Read the model definition and answer for the solid it produces. Units are mm, in the model's axes. Face numbers are marked on the shaded views. A direction names the side the tool comes from. Coordinates: 2 decimals unless noted, no trailing zeros. Write each loop counter-clockwise with the first axis right and the second up, starting at its lowest first coordinate (ties: lowest second). Pieces come first, ordered by that corner, then holes.
Item 1: A tool of negligible diameter and unlimited length cuts with its end or side. For the marked faces 4, 5 and 6, from which of +Z, -Z, +X, -X, +Y, -Y can it reach the whole face along a straight path? Write none if from no direction.
Item 2: Section D-D (z = -4) is taken. Give the vertices of the cut face in (x, y), then the cut area to 3 significant figures.
Item 3: Section B-B (y = 5.25) is taken. Give the vertices of the cut face in (x, z), then the cut area to 3 significant figures.
Item 4: Section C-C (x = 0) is taken. Give the vertices of the cut face in (y, z), then the cut area to 3 significant figures.
Item 5: Section A-A (z = -7) is taken. Give the vertices of the cut face in (x, y).
Item 6: Straight lines are drawn through the part: probe 1 along Z at (x, y) = (1.25, 8.5); probe 2 along X at (y, z) = (0, -6.1); probe 3 along Y at (x, z) = (0, -6.6). For each, find the intervals that lie inside material, in ascending order.
Item 7: Each of these flat-tipped pins is pushed along its axis until it touches: P1, Ø2, axis at x = 4, z = 0, coming from the +Y side; P2, Ø4, axis at y = -4, z = -6.5, coming from the -X side; P3, Ø1.5, axis at x = 7.5, z = -2, coming from the -Y side; P4, Ø1.5, axis at x = -0.5, y = -0.5, coming from the -Z side. Where does it stop, or does it pass through?
Item 8: Determine the mould class of the marked faces 1, 2 and 3 for opening direction X: released by +X, released by -X, zero draft, split by the parting line, or undercut.
from build123d import *

# Parameters (mm, degrees)
F0_R     = 10.5
F0_R_2   = 9
F0_R_3   = 3
F1_DEPTH = 1
F2_DEPTH = 5
F3_DEPTH = 0.1
F4_DEPTH = 0.1
F5_R     = 9
F6_DEPTH = 0.1
F7_R     = 1.5
F8_DEPTH = 4.5


with BuildPart() as f1:
    # F0 (on Top) → F1 (new body)
    with BuildSketch(Plane.XY):
        Circle(F0_R)
        Circle(F0_R_2, mode=Mode.SUBTRACT)
        Circle(F0_R_2)
        Circle(F0_R_3, mode=Mode.SUBTRACT)
        Circle(F0_R_3)
    extrude(amount=F1_DEPTH)

    # F0 (on Top) → F2 (join)
    with BuildSketch(Plane.XY):
        Circle(F0_R_3)
    extrude(amount=-F2_DEPTH)

    # F0 (on Top) → F3 (join)
    with BuildSketch(Plane.XY):
        Circle(F0_R_2)
        Circle(F0_R_3, mode=Mode.SUBTRACT)
    extrude(amount=F3_DEPTH)

    # F0 (on Top) → F4 (join)
    with BuildSketch(Plane.XY):
        Circle(F0_R_2)
        Circle(F0_R_3, mode=Mode.SUBTRACT)
    extrude(amount=-F4_DEPTH)

    # F5 (on face) → F6 (join)
    with BuildSketch(Plane.XY.offset(1)):
        Circle(F5_R)
    extrude(amount=F6_DEPTH)

    # F7 (on face) → F8 (join)
    with BuildSketch(Plane(origin=(0, 0, -5), x_dir=(1, 0, 0), z_dir=(0, 0, -1))):
        Polygon((1.668331337, -2.4933251994), (2.9934486311, 0.1981547201), (1.325117294, 2.6914799195), (-1.668331337, 2.4933251994), (-2.9934486311, -0.1981547201), (-1.325117294, -2.6914799195), align=None)
        Circle(F7_R, mode=Mode.SUBTRACT)
    extrude(amount=F8_DEPTH)


solid = f1.part
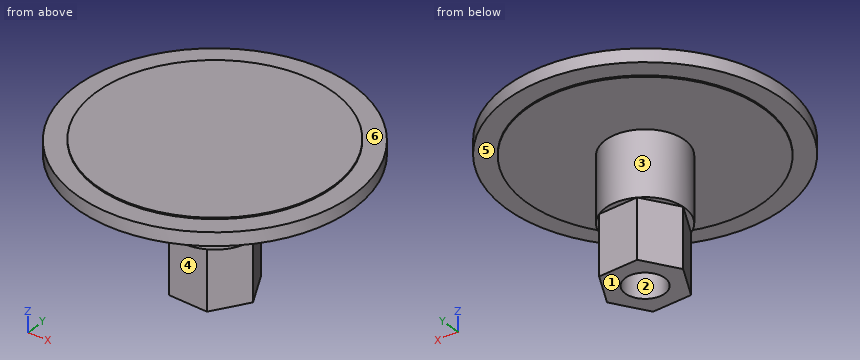
Established:
1. face 4: -Z, -X, -Y
1. face 5: -Z
1. face 6: +Z
2. outline: circle Ø6 at (0, 0)
2. area: 28.3 mm2
3. outline: (-9.09, 0) - (-7.31, 0) - (-7.31, -0.1) - (7.31, -0.1) - (7.31, 0) - (9.09, 0) - (9.09, 1) - (7.31, 1) - (7.31, 1.1) - (-7.31, 1.1) - (-7.31, 1) - (-9.09, 1) - close
3. area: 21.1 mm2
4. outline: (-10.5, 0) - (-9, 0) - (-9, -0.1) - (-3, -0.1) - (-3, -5) - (-2.6, -5) - (-2.6, -9.5) - (-1.5, -9.5) - (-1.5, -5) - (1.5, -5) - (1.5, -9.5) - (2.6, -9.5) - (2.6, -5) - (3, -5) - (3, -0.1) - (9, -0.1) - (9, 0) - (10.5, 0) - (10.5, 1) - (9, 1) - (9, 1.1) - (-9, 1.1) - (-9, 1) - (-10.5, 1) - close
4. area: 63.9 mm2
5. outline: (-2.99, 0.2) - (-1.67, -2.49) - (1.33, -2.69) - (2.99, -0.2) - (1.67, 2.49) - (-1.33, 2.69) - close; hole circle Ø3 at (0, 0)
6. probe 1: z = -0.1 to 1.1
6. probe 2: x = -2.9 to -1.5, 1.5 to 2.9
6. probe 3: y = -2.6 to -1.5, 1.5 to 2.6
7. P1: stops at y = 10.06
7. P2: stops at x = -1.91
7. P3: passes through
7. P4: stops at z = -5
8. face 1: zero draft
8. face 2: undercut
8. face 3: split by the parting line
